from build123d import *

# Parameters (mm, degrees)
F1_DEPTH    = 38.1
F2_T1_DEPTH = 53.6803294212


# Not quite as in the source:
# - a fillet or chamfer that OpenCascade refuses, or shapes differently, is made with other operations: its cross-section is extruded or revolved along the edge and cut away or added


with BuildPart() as f1:
    # F0 (on Top) → F1 (new body)
    with BuildSketch(Plane.XY):
        Polygon((-7.2168783649, -12.5), (7.2168783649, -12.5), (14.4337567297, 0), (28.8675134595, 0), (36.0843918244, 12.5), (28.8675134595, 25), (14.4337567297, 25), (7.2168783649, 12.5), (-7.2168783649, 12.5), (-14.4337567297, 0), align=None)
        Polygon((12.124355653, 0), (6.0621778265, -10.5), (-6.0621778265, -10.5), (-12.124355653, 0), (-6.0621778265, 10.5), (6.0621778265, 10.5), (9.5262794416, 12.5), (15.5884572681, 23), (27.7128129211, 23), (33.7749907476, 12.5), (27.7128129211, 2), (15.5884572681, 2), align=None, mode=Mode.SUBTRACT)
    extrude(amount=F1_DEPTH)

    # F2: chamfer of 3 on 4 edges, made by hand

    # F2_s2 → F2_t1 (cut)
    with BuildSketch(Plane.XY.offset(-7.7901647106)):
        Polygon((3.0621778265, 10.5), (8.6602540378, 12), (6.0621778265, 10.5), align=None)
        Polygon((6.9282032303, 11), (11.0262794416, 15.0980762114), (9.5262794416, 12.5), align=None)
        Polygon((14.7224318643, 1.5), (10.624355653, -2.5980762114), (12.124355653, 0), align=None)
        Polygon((18.5884572681, 2), (12.9903810568, 0.5), (15.5884572681, 2), align=None)
    extrude(amount=F2_T1_DEPTH, mode=Mode.SUBTRACT)


solid = f1.part
CAD build for the part. Positions are in the model's coordinates, mm. A direction names the side the tool comes from. Coordinates: 2 decimals unless noted, no trailing zeros. Write each loop counter-clockwise with the first axis right and the second up, starting at its lowest first coordinate (ties: lowest second). Pieces come first, ordered by that corner, then holes. Notation, with made-up numbers: (-5, 73) - (47, 73) arc R14 cw to (47, 83) - close; hole circle Ø1 at (-18.5, -29.5). An arc over 180 degrees is marked (long way). Use a Markdown table: item, result. Add a question column.
Item 1: Band-saw the part on A-A, the plane x = -4.5. Give the cut face in (y, z).
Item 2: Band-saw the part on B-B, the plane z = 4. Give the cut face in (x, y) (3 decimals).
Item 3: Flat gauge pins, fed straight in: pin 1 (6 mm diameter, centred on x = 23.5, z = 25.5, fed in from -Y); pin 2 (12 mm diameter, centred on y = 21, z = 6.5, fed in from +X); pin 3 (7 mm diameter, centred on x = -0.5, z = 15.5, fed in from +Y). Where does each tip first touch, or does it go through?
Item 4: Drill centre lines: L1, parallel to Y at x = 27.5, z = 12; L2, parallel to Y at x = 3.5, z = 11; L3, parallel to X at y = -0.5, z = 34. Where is each one in solid material? Low to high. Write a range as from..to.
Item 5: Mould opens along X. For faces 4 (the face through (0, -12.5, 19)), 5 (the face through (32.425, 6.163, 18.783)), 6 (the face through (-9.136, 5.177, 18.783)) say: pulls with the +X half, pulls with the -X half, needs draft (parallel to the pull), parting line crosses it, or undercut.
Item 6: Band-saw the part on C-C, the plane y = 17. Give the cut face in (x, z).
Item 7: 3-axis set-ups, long thin cutter, end or side, ignore diameter. For faces 1 (the face through (22, 0, 19)), 2 (the face through (32.53, 18.66, 18.78)), 3 (the face through (16.322, 1.393, 18.783)): which of +Z, -Z, +X, -X, +Y, -Y reach the whole face in a straight line?
Numbers:
| question | item | result |
|---|---|---|
| 1 | outline | (-12.5, 0) - (-10.5, 0) - (-10.5, 38.1) - (-12.5, 38.1) - close; (10.5, 0) - (12.5, 0) - (12.5, 38.1) - (10.5, 38.1) - close |
| 2 | outline | (-14.434, 0) - (-7.217, -12.5) - (7.217, -12.5) - (14.434, 0) - (28.868, 0) - (36.084, 12.5) - (28.868, 25) - (14.434, 25) - (7.217, 12.5) - (-7.217, 12.5) - close; hole (-12.124, 0) - (-6.062, -10.5) - (6.062, -10.5) - (10.624, -2.598) - (13.99, 0.768) - (18.588, 2) - (27.713, 2) - (33.775, 12.5) - (27.713, 23) - (15.588, 23) - (11.026, 15.098) - (7.66, 11.732) - (3.062, 10.5) - (-6.062, 10.5) - close |
| 3 | pin 1 | y = 0 |
| 3 | pin 2 | x = 34.64 |
| 3 | pin 3 | y = 12.5 |
| 4 | L1 | 0..2, 23..25 |
| 4 | L2 | -12.5..-10.5, 10.62..12.5 |
| 4 | L3 | -14.15..-11.84, 12.72..14.15 |
| 5 | face 4 | needs draft |
| 5 | face 5 | pulls with the +X half |
| 5 | face 6 | undercut |
| 6 | outline | (9.81, 0) - (12.12, 0) - (12.12, 38.1) - (9.81, 38.1) - close; (31.18, 0) - (33.49, 0) - (33.49, 38.1) - (31.18, 38.1) - close |
| 7 | face 1 | +Z, -Z, +X, -Y |
| 7 | face 2 | +Z, -Z, +X, +Y |
| 7 | face 3 | +Z, -Z |
